Input: part model. Units: mm. Frame: model coordinates. A direction names the side the tool comes from. Coordinates: 2 decimals unless noted, no trailing zeros. Write each loop counter-clockwise with the first axis right and the second up, starting at its lowest first coordinate (ties: lowest second). Pieces come first, ordered by that corner, then holes.
1) Section query B-B (z = -22.5). Output: boundary loops of the cut face in (x, y), then the cut area to 3 significant figures.
2) Draft query along Z for faces 1 (the flat face through (74, 4, 0)), 2 (the flat face through (76, 4, -200)), 3 (the flat face through (75, 4, -90)), 4 (the flat face through (74, 0, -101)). Return one class per face: pulls with the +Z half, pulls with the -Z half, needs draft (parallel to the pull), parting line crosses it, or undercut.
3) Section query D-D (x = 60.5). Output: boundary loops of the cut face in (y, z).
4) Pin query (flat end, axial travel): pin 1 Ø4 at (x, z) = (15, -196.25) entering from -Y. Return the tip coordinate at first contact, or that it passes through.
5) Section query A-A (x = 15). Output: boundary loops of the cut face in (y, z).
6) Set-up query: faces 5 (the flat face through (150, 4, -99)), 6 (the flat face through (55, 4, -95)). Return all of +Z, -Z, +X, -X, +Y, -Y with unobstructed straight access to the full face (end or side cutting, diameter ignored); none if empty.
7) Line query: L1, parallel to Z at x = 15, y = 2; L2, parallel to X at y = 5, z = -50; L3, parallel to X at y = 4.5, z = -196.25. Output: solid intervals per line, ascending.
8) Section query C-C (y = 1.5). State how many separate pieces and enclosed holes the cut face has, then the cut area to 3 significant figures.
from build123d import *

# Parameters (mm, degrees)
CROQUIS1_R              = 0.6
CROQUIS1_R_2            = 6
SALIENTE_EXTRUIR2_DEPTH = 7.5
CROQUIS4_R              = 2.5
CORTAR_EXTRUIR1_DEPTH   = 7.5


with BuildPart() as part:
    # Croquis1 → Saliente-Extruir2 (new body)
    with BuildSketch(Plane(origin=(0, 0, 0), x_dir=(1, 0, 0), z_dir=(0, 1, 0))):
        Polygon((0, 200), (0, 100), (55, 100), (95, 100), (150, 100), (150, 200), align=None)
        Polygon((55, 100), (0, 100), (0, 0), (150, 0), (150, 100), (95, 100), (95, 90), (75, 90), (55, 90), align=None)
        with Locations((75, 40)):
            Circle(CROQUIS1_R, mode=Mode.SUBTRACT)
        with Locations((65, 50)):
            Circle(CROQUIS1_R, mode=Mode.SUBTRACT)
        with Locations((75, 50)):
            Circle(CROQUIS1_R_2, mode=Mode.SUBTRACT)
        with Locations((75, 60)):
            Circle(CROQUIS1_R, mode=Mode.SUBTRACT)
        with Locations((85, 50)):
            Circle(CROQUIS1_R, mode=Mode.SUBTRACT)
    extrude(amount=SALIENTE_EXTRUIR2_DEPTH)

    # Croquis4 → Cortar-Extruir1 (cut)
    with BuildSketch(Plane.XZ):
        with Locations((135, -3.75)):
            Circle(CROQUIS4_R)
        with Locations((146.25, -22.5)):
            Circle(CROQUIS4_R)
        with Locations((3.75, -22.5)):
            Circle(CROQUIS4_R)
        with Locations((15, -3.75)):
            Circle(CROQUIS4_R)
        with Locations((146.25, -177.5)):
            Circle(CROQUIS4_R)
        with Locations((135, -196.25)):
            Circle(CROQUIS4_R)
        with Locations((3.75, -177.5)):
            Circle(CROQUIS4_R)
        with Locations((15, -196.25)):
            Circle(CROQUIS4_R)
    extrude(amount=-CORTAR_EXTRUIR1_DEPTH, mode=Mode.SUBTRACT)


solid = part.part
Answer:
1. outline: (0, 0) - (1.25, 0) - (1.25, 7.5) - (0, 7.5) - close; (6.25, 0) - (143.75, 0) - (143.75, 7.5) - (6.25, 7.5) - close; (148.75, 0) - (150, 0) - (150, 7.5) - (148.75, 7.5) - close
1. area: 1,050 mm2
2. face 1: pulls with the +Z half
2. face 2: pulls with the -Z half
2. face 3: undercut
2. face 4: needs draft
3. outline: (0, -200) - (7.5, -200) - (7.5, -100) - (0, -100) - close; (0, -90) - (7.5, -90) - (7.5, 0) - (0, 0) - close
4. pin 1: passes through
5. outline: (0, -200) - (7.5, -200) - (7.5, -198.75) - (0, -198.75) - close; (0, -193.75) - (7.5, -193.75) - (7.5, -6.25) - (0, -6.25) - close; (0, -1.25) - (7.5, -1.25) - (7.5, 0) - (0, 0) - close
6. face 5: +Z, -Z, +X, +Y, -Y
6. face 6: +Y, -Y
7. L1: z = -200 to -198.75, -193.75 to -6.25, -1.25 to 0
7. L2: x = 0 to 64.4, 65.6 to 69, 81 to 84.4, 85.6 to 150
7. L3: x = 0 to 12.5, 17.5 to 132.5, 137.5 to 150
8. separate pieces: 1
8. enclosed holes: 14
8. area: 29,300 mm2
